```python
from build123d import *

# Parameters (mm, degrees)
SKETCH2_W           = 6
SKETCH2_H           = 8.3
SHELL1_T            = -0.3
SKETCH5_R           = 1.25
CUT_EXTRUDE1_DEPTH  = 10
FILLET1_R           = 1
FILLET2_R           = 0.1
CHAMFER1_SIZE       = 0.5
BOSS_EXTRUDE1_DEPTH = 1


with BuildPart() as part:
    # Sketch2 → Revolve1 (revolve)
    with BuildSketch(Plane.XY):
        with Locations((-3.662621359, 4.15)):
            Rectangle(SKETCH2_W, SKETCH2_H)
    revolve(axis=Axis((0, 0, 0), (-1, 0, 0)))

    # Sketch3 → Revolve2 (revolve)
    with BuildSketch(Plane.XY, mode=Mode.PRIVATE) as revolve2_sk:
        Polygon((1.337378641, 7.188452486), (-0.662621359, 7.328306109), (-0.662621359, 5.688452486), (1.337378641, 5.688452486), align=None)
    revolve(revolve2_sk.sketch.rotate(Axis((-0.662621359, 5.688452486, 0), (1, 0, 0)), 180), axis=Axis((-0.662621359, 5.688452486, 0), (1, 0, 0)))

    # Shell1
    shell1_openings = [part.faces().sort_by_distance(p)[0] for p in [
        (-6.662621359, 0, 0),
    ]]
    offset(amount=SHELL1_T, openings=shell1_openings, kind=Kind.INTERSECTION)

    # Sketch5 → Cut-Extrude1 (cut)
    with BuildSketch(Plane(origin=(1.337378641, 0, 0), x_dir=(0, 0, -1), z_dir=(1, 0, 0))):
        with Locations((0, 5.688452486)):
            Circle(SKETCH5_R)
    extrude(amount=-CUT_EXTRUDE1_DEPTH, mode=Mode.SUBTRACT)

    # Fillet1
    fillet1_edges = [part.edges().sort_by_distance(p)[0] for p in [
        (-0.662621359, -8.3, 0),
    ]]
    fillet(fillet1_edges, radius=FILLET1_R)

    # Fillet2
    fillet2_edges = [part.edges().sort_by_distance(p)[0] for p in [
        (1.337378641, 7.188452486, 0),
    ]]
    fillet(fillet2_edges, radius=FILLET2_R)

    # Chamfer1
    # the kernel refuses this chamfer: 0.5 mm, written as the material it takes off along each edge
    with BuildSketch(Plane(origin=(-6.662621359, 0, 0), x_dir=(0, 1, 0), z_dir=(0, 0, -1))) as chamfer1_piece_1:
        Polygon((8 + CHAMFER1_SIZE, 0), (8, CHAMFER1_SIZE), (8, 0), align=None)
    revolve(axis=Axis((-6.662621359, 0, 0), (1, 0, 0)), mode=Mode.SUBTRACT)

    # Sketch6 → Boss-Extrude1 (add, symmetric)
    with BuildSketch(Plane.XY):
        with BuildLine():
            Line((-4.927907027, 8.3), (-4.927907027, 8.730333701))
            ThreePointArc((-4.927907027, 8.730333701), (-4.212236683, 10.597628426), (-2.431874659, 11.508279126))
            ThreePointArc((-2.431874659, 11.508279126), (-2.223300905, 11.440869947), (-2.134041341, 11.2406707))
            Line((-2.134041341, 11.2406707), (-2.134041341, 8.115869894))
            Line((-2.134041341, 8.115869894), (-4.927907027, 8.115869894))
            Line((-4.927907027, 8.115869894), (-4.927907027, 7.714440325))
            Line((-4.927907027, 7.714440325), (-4.927907027, 8.3))
        make_face()
        with BuildLine():
            Line((-4.467319737, 8.752860733), (-2.584041341, 8.752860733))
            ThreePointArc((-2.584041341, 8.752860733), (-2.442619985, 8.811439376), (-2.384041341, 8.952860733))
            Line((-2.384041341, 8.952860733), (-2.384041341, 11.030595936))
            ThreePointArc((-2.384041341, 11.030595936), (-2.456918607, 11.184997395), (-2.622439446, 11.226875292))
            ThreePointArc((-2.622439446, 11.226875292), (-4.018863264, 10.438753715), (-4.666416333, 8.971848769))
            ThreePointArc((-4.666416333, 8.971848769), (-4.61530218, 8.818320046), (-4.467319737, 8.752860733))
        make_face(mode=Mode.SUBTRACT)
    extrude(amount=BOSS_EXTRUDE1_DEPTH, both=True)


solid = part.part
```
The listing builds one solid part. Answer for the finished solid, in the listing's coordinates (mm). A direction names the side the tool comes from. Give positions to 0.01 mm unless a question says otherwise; leave off trailing zeros. Order: outer loops, then holes, each group sorted by start corner. A loop starts at its lowest first (then second) coordinate and runs counter-clockwise, first axis right, second up.
Item 1: Find the intervals of material crossed by probe 1 along Z at (x, y) = (-3.55, 0); probe 2 along X at (y, z) = (-2.75, -4); probe 3 along Y at (x, z) = (-5.5, -6.75), in increasing order.
From the geometry:
probe 1: z = -8.3 to -8, 8 to 8.3
probe 2: x = -0.96 to -0.66
probe 3: y = -4.83 to -4.29, 4.29 to 4.83
Item 2: For a pull along X with two mould halves and no side action, classify faces 6 (the face through (-3.4, 8.5, 1)), 7 (the face through (-4, 10.46, 0.01)), 8 (the face through (-0.01, 6.98, -0.06)) as pulls with the +X half, pulls with the -X half, needs draft (parallel to the pull), parting line crosses it, or undercut.
From the geometry:
face 6: needs draft
face 7: undercut
face 8: pulls with the -X half
Item 3: Which of the six approach directions +Z, -Z, +X, -X, +Y, -Y give full straight-line access (tool end or side, diameter ignored) to faces 1 (the face through (-4, 8.753, 0)), 2 (the face through (0.98, 6.93, 0.16)), 3 (the face through (-3.4, 8.5, -1)), 4 (the face through (-3.53, -1.73, 7.81)), 5 (the face through (0.489, 7.246, -0.069))?
From the geometry:
face 1: +Z, -Z
face 2: +X, -X
face 3: -Z, +X, -X, +Y
face 4: -X
face 5: +X
Item 4: Given pin 1 Ø1 at (x, z) = (-2.5, -3.5) entering from -Y; pin 2 Ø0.5 at (y, z) = (8.5, 0) entering from -X; pin 3 Ø0.6 at (y, z) = (9.5, 0) entering from -X; pin 4 Ø4 at (y, z) = (-3, 4) entering from -X, each flat-ended and moving along its own axis, determine where each tip first touches the part or whether it passes through.
From the geometry:
pin 1: stops at y = -7.74
pin 2: stops at x = -6.46
pin 3: stops at x = -4.89
pin 4: stops at x = -0.96
Item 5: The part is cut by section A-A, the plane y = 0. Give the vertices of the cut face in (x, z).
From the geometry:
outline: (-6.46, -8.3) - (-1.66, -8.3) arc R1 ccw to (-0.66, -7.3) - (-0.66, 7.3) arc R1 ccw to (-1.66, 8.3) - (-6.46, 8.3) - (-6.16, 8) - (-0.96, 8) - (-0.96, -8) - (-6.16, -8) - close
Item 6: The part is cut by section B-B, the plane z = 0.75. Count the separate pieces of the cut face and the enclosed holes in it, and give its area (3 significant figures).
From the geometry:
separate pieces: 2
enclosed holes: 1
area: 11.5 mm2
